from build123d import *

# Parameters (mm, degrees)
BOSS_EXTRUDE1_DEPTH            = 3.175
M4_CLEARANCE_HOLE1_D           = 4.5
M4_CLEARANCE_HOLE1_CSINK_D     = 4.55
M4_CLEARANCE_HOLE1_CSINK_ANGLE = 90
M8_CLEARANCE_HOLE1_AT_2_COUNT  = 2
M8_CLEARANCE_HOLE1_AT_2_PITCH  = 84
SKETCH9_R                      = 21.275
CENTER_HOLE_DEPTH              = 87.427675689


with BuildPart() as part:
    # Sketch1 → Boss-Extrude1 (new body)
    with BuildSketch(Plane.XY):
        Polygon((-69.85, 48.26), (-69.85, 38.1), (-69.85, -38.1), (69.85, -38.1), (69.85, 38.1), (69.85, 50.8), align=None)
    extrude(amount=BOSS_EXTRUDE1_DEPTH)

    # M4 Clearance Hole1 (through all)
    with Locations(Plane.XY.offset(3.175)):
        with Locations((-61.9125, -30.1625), (0, -30.1625), (61.9125, -30.1625), (61.9125, 30.1625), (61.9125, 0), (0, 30.1625), (-61.9125, 30.1625), (-61.9125, 0)):
            CounterSinkHole(M4_CLEARANCE_HOLE1_D / 2, M4_CLEARANCE_HOLE1_CSINK_D / 2, counter_sink_angle=M4_CLEARANCE_HOLE1_CSINK_ANGLE)

    # Sketch11 → M8 Clearance Hole1 (revolve, cut)
    with BuildSketch(Plane(origin=(-42, 0, 3.175), x_dir=(0, -1, 0), z_dir=(1, 0, 0))):
        Polygon((0, 0), (0, 3.175), (4.5, 3.175), (4.5, 0.025), (4.525, 0), align=None)
    m8_clearance_hole1 = revolve(axis=Axis((-42, 0, 9.525), (0, 0, -1)), mode=Mode.SUBTRACT)

    # M8 Clearance Hole1 at 2: M8 Clearance Hole1 ×2
    with Locations(*[(i * M8_CLEARANCE_HOLE1_AT_2_PITCH, 0, 0) for i in range(1, M8_CLEARANCE_HOLE1_AT_2_COUNT)]):
        add(m8_clearance_hole1, mode=Mode.SUBTRACT)

    # Sketch9 → Center Hole (cut, through all)
    with BuildSketch(Plane.XY.offset(3.175)):
        Circle(SKETCH9_R)
    extrude(amount=-CENTER_HOLE_DEPTH, mode=Mode.SUBTRACT)


solid = part.part
Can you work these out from the model? Positions are in its coordinate system, mm. Give positions to 0.01 mm unless a question says otherwise; leave off trailing zeros. Loops run counter-clockwise (first coordinate to the right, second up) from the corner with the lowest first, then second, coordinate; pieces in that order, holes last. Notation, with made-up numbers: (77.5, 48.25) -> (121.5, 48.25) arc R4 cw to (121.5, 53.25) -> close; hole circle Ø10 at (-36.75, 29). An arc over 180 degrees is marked (long way). Return JSON: item names as keys, results as strings.
Q1. We'd pull the mould along X, two halves only. Please class faces 1 (the face through (-1.21, -28.265, 1.553)), 2 (the face through (69.85, 6, 2)), 3 (the face through (-1, -38.1, 2)), 4 (the face through (-69.85, 6, 2)): released by +X, released by -X, zero draft, split by the parting line, or undercut.
Checks:
{"face 1": "undercut", "face 2": "released by +X", "face 3": "zero draft", "face 4": "released by -X"}
Q2. I want a section at D-D, the plane x = 42. List the corners of the cut face in (y, z) for me (3 decimals), then the cut area to 3 significant figures.
Checks:
{"outline": "(-38.1, 0) -> (-4.5, 0) -> (-4.5, 3.15) -> (-4.525, 3.175) -> (-38.1, 3.175) -> close; (4.5, 0) -> (50.294, 0) -> (50.294, 3.175) -> (4.525, 3.175) -> (4.5, 3.15) -> close", "area": "252 mm2"}
Q3. I need wall thicknesses on probe 1 along X at (y, z) = (-1, 1.8); probe 2 along X at (y, z) = (-31, 1.5); probe 3 along Y at (x, z) = (0, 0.8) (1 decimal). Which ranges of each line are inside material? Lowest first, please.
Checks:
{"probe 1": "x = -69.85 to -63.93, -59.9 to -46.39, -37.61 to -21.25, 21.25 to 37.61, 46.39 to 59.9, 63.93 to 69.85", "probe 2": "x = -69.85 to -64, -59.82 to -2.09, 2.09 to 59.82, 64 to 69.85", "probe 3": "y = -38.1 to -32.4, -27.9 to -21.3, 21.3 to 27.9, 32.4 to 49.5"}
Q4. I want a section at C-C, the plane y = 11.5. List the corners of the cut face in (x, z) for me (3 decimals).
Checks:
{"outline": "(-69.85, 0) -> (-17.899, 0) -> (-17.899, 3.175) -> (-69.85, 3.175) -> close; (17.899, 0) -> (69.85, 0) -> (69.85, 3.175) -> (17.899, 3.175) -> close"}
Q5. I want a section at A-A, the plane y = 0. Count the separate pieces of the cut face and the enclosed holes in it, then the cut area to 3 significant figures.
Checks:
{"separate pieces": "6", "enclosed holes": "0", "area": "223 mm2"}
Q6. For pin 1 Ø1 at (x, z) = (-21, 2.5) entering from +Y; pin 2 Ø1.5 at (x, z) = (-7, 0.5) entering from +Y, each with a flat end and sliding along its axis, tell me the tip position at first contact or that it passes through.
Checks:
{"pin 1": "stops at y = 49.16", "pin 2": "stops at y = 49.42"}
